Geometry: final body of the model. Coordinates: model frame, mm. Face numbers are marked on the shaded views. A direction names the side the tool comes from. Coordinates: 2 decimals unless noted, no trailing zeros. Loops run counter-clockwise (first coordinate to the right, second up) from the corner with the lowest first, then second, coordinate; pieces in that order, holes last. Notation, with made-up numbers: (9.5, 31.25) - (32.5, 31.25) arc R3 ccw to (32.5, 36.25) - close; hole circle Ø2 at (20.5, 8.25). An arc over 180 degrees is marked (long way). Answer in a Markdown table with one row per item.
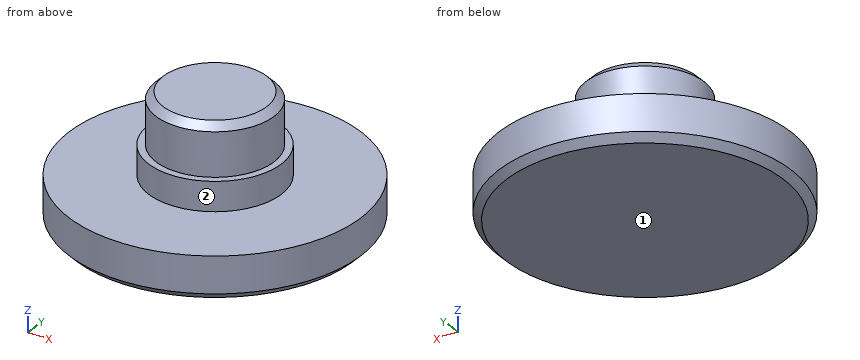
from build123d import *

# Parameters (mm, degrees)
F0_R     = 10
F1_DEPTH = 3
F2_R     = 4.05
F3_DEPTH = 5.5
F4_SIZE  = 0.5
F5_R     = 4.55
F6_DEPTH = 2


with BuildPart() as f1:
    # F0 (on Top) → F1 (new body)
    with BuildSketch(Plane.XY):
        Circle(F0_R)
    extrude(amount=F1_DEPTH)

    # F2 (on face) → F3 (join)
    with BuildSketch(Plane.XY.offset(3)):
        Circle(F2_R)
    extrude(amount=F3_DEPTH)

    # F4
    f4_edges = [f1.edges().sort_by_distance(p)[0] for p in [
        (-4.05, 0, 8.5),
        (-10, 0, 0),
    ]]
    chamfer(f4_edges, length=F4_SIZE)

    # F5 (on face) → F6 (join)
    with BuildSketch(Plane.XY.offset(3)):
        Circle(F5_R)
    extrude(amount=F6_DEPTH)


solid = f1.part
(1) Cut plane A-A on y = 0. Output: boundary loops of the cut face in (x, z), then the cut area to 3 significant figures.
Verdict:
| item | result |
|---|---|
| outline | (-10, 0.5) - (-9.5, 0) - (9.5, 0) - (10, 0.5) - (10, 3) - (4.55, 3) - (4.55, 5) - (4.05, 5) - (4.05, 8) - (3.55, 8.5) - (-3.55, 8.5) - (-4.05, 8) - (-4.05, 5) - (-4.55, 5) - (-4.55, 3) - (-10, 3) - close |
| area | 106 mm² |
(2) Ray query, probe 1 along Z at (x, y) = (1, -5.75); probe 2 along Y at (x, z) = (0, 4.5); probe 3 along X at (y, z) = (0.25, 6.25). Return the intervals inside material, ascending.
Verdict:
| item | result |
|---|---|
| probe 1 | z = 0 to 3 |
| probe 2 | y = -4.55 to 4.55 |
| probe 3 | x = -4.04 to 4.04 |
(3) Cut plane C-C on z = 1.25. Output: boundary loops of the cut face in (x, y), then the cut area to 3 significant figures.
Verdict:
| item | result |
|---|---|
| outline | circle Ø20 at (0, 0) |
| area | 314 mm² |
(4) First-contact query: pin 1 Ø1.5 at (x, z) = (3, 4) entering from -Y; pin 2 Ø1 at (y, z) = (6.5, 4.5) entering from -X. Flat tips, straight axial feed; report the tip coordinate or a pass-through.
Verdict:
| item | result |
|---|---|
| pin 1 | stops at y = -3.95 |
| pin 2 | passes through |
(5) Access query for the marked faces 1 and 2. Directions: +Z, -Z, +X, -X, +Y, -Y. A direction counts if a zero-diameter tool reaches every point of the face in a straight line with its end or side. Return the directions, or none.
Verdict:
| item | result |
|---|---|
| face 1 | -Z, +X, -X, +Y, -Y |
| face 2 | +Z |
(6) Cut plane D-D on z = 6.5. Output: boundary loops of the cut face in (x, y).
Verdict:
| item | result |
|---|---|
| outline | circle Ø8.1 at (0, 0) |
